Verification items for the finished model (mm, model axes). Face numbers are marked on the shaded views. A direction names the side the tool comes from. Round coordinates to 2 decimals unless told otherwise and drop trailing zeros. Order: outer loops, then holes, each group sorted by start corner. A loop starts at its lowest first (then second) coordinate and runs counter-clockwise, first axis right, second up. Notation, with made-up numbers: M 81.25,61.25 L 91.25,61.25 A27 cw 91.25,92.25 Z; hole C -22.75,-25 d10. An arc over 180 degrees is marked long. Use CSV: the item, a comma, the result in double quotes. Start each with the question number.
Q1. Set-up check for the marked faces 5, 6 and 7: record each of +Z, -Z, +X, -X, +Y, -Y from which the full face is reachable in a straight line by a thin tool's end or side.
Q2. Sectioned sample at B-B (x = 41). Enter the section's corners in (y, z), and give its area (3 significant figures).
Q3. Sectioned sample at C-C (z = 6). Enter the section's corners in (x, y) (3 decimals), and give its area (3 significant figures).
Q4. Mould release check, pull along X, two halves, no side actions. Record for the marked faces 1, 2, 3 and 4: +X half, -X half, draft (parallel to the pull), parting line (faces both ways), or undercut.
Q5. Sectioned sample at D-D (y = 43). Enter the section's corners in (x, z).
Q6. Sectioned sample at A-A (y = 17). Enter the section's corners in (x, z) (3 decimals).
Q7. Scan lines: line 1 (Z direction, x = -88, y = 8.5); line 2 (Z direction, x = -26.5, y = 17); line 3 (X direction, y = -8.5, z = 23). Record each from-to range of solid material in increasing order.
Q8. Gauge pin test, flat ends, axial feed: pin 1 Ø12 at (x, z) = (-36, 21.5) entering from +Y; pin 2 Ø0.6 at (x, z) = (98, 33) entering from +Y; pin 3 Ø1.5 at (x, z) = (60.5, 18.5) entering from +Y. Record the tip position at first contact, or that the pin passes through.
```python
from build123d import *

# Parameters (mm, degrees)
SKETCH2_W                = 198
SKETCH2_H                = 78
BOSS_EXTRUDE1_DEPTH      = 50
BOSS_EXTRUDE1_DEPTH_BACK = 15
SHELL1_T                 = -2
BOSS_EXTRUDE2_REACH      = 198
SKETCH3_W                = 2.5
SKETCH3_H                = 2
CUT_EXTRUDE1_REACH       = 4
CROQUIS1_W               = 35.265
CROQUIS1_H               = 26
SALIENTE_EXTRUIR1_DEPTH  = 38.9
CORTAR_EXTRUIR1_DEPTH    = 2
CORTAR_EXTRUIR2_DEPTH    = 30
CROQUIS5_W               = 26
CROQUIS5_H               = 15
CORTAR_EXTRUIR3_DEPTH    = 35.265
CROQUIS6_W               = 12
CROQUIS6_H               = 3
SALIENTE_EXTRUIR2_DEPTH  = 3
CROQUIS7_W               = 26
CROQUIS7_H               = 15
CORTAR_EXTRUIR4_DEPTH    = 35.265


with BuildPart() as part:
    # Sketch2 → Boss-Extrude1 (new body, two sides)
    with BuildSketch(Plane(origin=(0, 0, 0), x_dir=(1, 0, 0), z_dir=(0, 1, 0))) as boss_extrude1_sk:
        Rectangle(SKETCH2_W, SKETCH2_H)
    extrude(amount=BOSS_EXTRUDE1_DEPTH)
    extrude(boss_extrude1_sk.sketch, amount=-BOSS_EXTRUDE1_DEPTH_BACK)

    # Shell1
    shell1_openings = [part.faces().sort_by_distance(p)[0] for p in [
        (0, 50, 0),
    ]]
    offset(amount=SHELL1_T, openings=shell1_openings, kind=Kind.INTERSECTION)

    # Sketch3 → Boss-Extrude2 (add, up to next)
    with BuildSketch(Plane(origin=(-97, 0, 0), x_dir=(0, 0, -1), z_dir=(1, 0, 0)), mode=Mode.PRIVATE) as boss_extrude2_sk1:
        with Locations((-35.75, 49)):
            Rectangle(SKETCH3_W, SKETCH3_H)
    boss_extrude2_tool1 = extrude(boss_extrude2_sk1.sketch, amount=BOSS_EXTRUDE2_REACH, mode=Mode.PRIVATE) - part.part
    add(boss_extrude2_tool1.solids().sort_by_distance((-97, 49, 35.75))[0])
    # Sketch3 → Boss-Extrude2 (add, up to next)
    with BuildSketch(Plane(origin=(-97, 0, 0), x_dir=(0, 0, -1), z_dir=(1, 0, 0)), mode=Mode.PRIVATE) as boss_extrude2_sk2:
        with Locations((35.75, 49)):
            Rectangle(SKETCH3_W, SKETCH3_H)
    boss_extrude2_tool2 = extrude(boss_extrude2_sk2.sketch, amount=BOSS_EXTRUDE2_REACH, mode=Mode.PRIVATE) - part.part
    add(boss_extrude2_tool2.solids().sort_by_distance((-97, 49, -35.75))[0])

    # Sketch4 → Cut-Extrude1 (cut, up to next)
    with BuildSketch(Plane.ZY.offset(-97), mode=Mode.PRIVATE) as cut_extrude1_sk1:
        Polygon((-37, 48), (-37, 45), (-31.5, 45), (-31.5, 50), (-34.5, 50), (-34.5, 48), align=None)
    cut_extrude1_tool1 = extrude(cut_extrude1_sk1.sketch, amount=-CUT_EXTRUDE1_REACH, mode=Mode.PRIVATE) & part.part
    add(cut_extrude1_tool1.solids().sort_by_distance((97, 47.166667, -33.916667))[0], mode=Mode.SUBTRACT)
    # Sketch4 → Cut-Extrude1 (cut, up to next)
    with BuildSketch(Plane.ZY.offset(-97), mode=Mode.PRIVATE) as cut_extrude1_sk2:
        Polygon((34.5, 48), (37, 48), (37, 45), (31.5, 45), (31.5, 50), (34.5, 50), align=None)
    cut_extrude1_tool2 = extrude(cut_extrude1_sk2.sketch, amount=-CUT_EXTRUDE1_REACH, mode=Mode.PRIVATE) & part.part
    add(cut_extrude1_tool2.solids().sort_by_distance((97, 47.166667, 33.916667))[0], mode=Mode.SUBTRACT)

    # Croquis1 → Saliente-Extruir1 (add)
    with BuildSketch(Plane(origin=(0, -13, 0), x_dir=(1, 0, 0), z_dir=(0, 1, 0))):
        with Locations((79.3675, -16.5)):
            Rectangle(CROQUIS1_W, CROQUIS1_H)
    saliente_extruir1 = extrude(amount=SALIENTE_EXTRUIR1_DEPTH)

    # Simetría1: Saliente-Extruir1 across plane
    add(saliente_extruir1.mirror(Plane(origin=(0, 0, 0), x_dir=(0, 0, 1), z_dir=(1, 0, 0))))

    # Croquis2 → Cortar-Extruir1 (cut)
    with BuildSketch(Plane(origin=(0, 25.9, 0), x_dir=(1, 0, 0), z_dir=(0, 1, 0))):
        with BuildLine():
            Line((82.41, -12.375), (82.41, -20.625))
            ThreePointArc((82.41, -20.625), (79.235, -23.8), (76.06, -20.625))
            Line((76.06, -20.625), (76.06, -12.375))
            ThreePointArc((76.06, -12.375), (79.235, -9.2), (82.41, -12.375))
        make_face()
    cortar_extruir1 = extrude(amount=-CORTAR_EXTRUIR1_DEPTH, mode=Mode.SUBTRACT)

    # Simetría2: Cortar-Extruir1 across plane
    add(cortar_extruir1.mirror(Plane(origin=(0, 0, 0), x_dir=(0, 0, 1), z_dir=(1, 0, 0))), mode=Mode.SUBTRACT)

    # Croquis3 → Cortar-Extruir2 (cut)
    with BuildSketch(Plane(origin=(0, 23.9, 0), x_dir=(1, 0, 0), z_dir=(0, 1, 0))):
        with BuildLine():
            Line((80.835, -13.2), (80.835, -19.8))
            ThreePointArc((80.835, -19.8), (79.235, -21.4), (77.635, -19.8))
            Line((77.635, -19.8), (77.635, -13.2))
            ThreePointArc((77.635, -13.2), (79.235, -11.6), (80.835, -13.2))
        make_face()
    cortar_extruir2 = extrude(amount=-CORTAR_EXTRUIR2_DEPTH, mode=Mode.SUBTRACT)

    # Simetría3: Cortar-Extruir2 across plane
    add(cortar_extruir2.mirror(Plane(origin=(0, 0, 0), x_dir=(0, 0, 1), z_dir=(1, 0, 0))), mode=Mode.SUBTRACT)

    # Croquis5 → Cortar-Extruir3 (cut)
    with BuildSketch(Plane.ZY.offset(-61.735)):
        with Locations((16.5, -5.5)):
            Rectangle(CROQUIS5_W, CROQUIS5_H)
    extrude(amount=-CORTAR_EXTRUIR3_DEPTH, mode=Mode.SUBTRACT)

    # Croquis6 → Saliente-Extruir2 (add)
    with BuildSketch(Plane.ZY.offset(-61.735)):
        with Locations((16.5, 3.5)):
            Rectangle(CROQUIS6_W, CROQUIS6_H)
    saliente_extruir2 = extrude(amount=SALIENTE_EXTRUIR2_DEPTH)

    # Croquis7 → Cortar-Extruir4 (cut)
    with BuildSketch(Plane(origin=(-61.735, 0, 0), x_dir=(0, 0, -1), z_dir=(1, 0, 0))):
        with Locations((-16.5, -5.5)):
            Rectangle(CROQUIS7_W, CROQUIS7_H)
    extrude(amount=-CORTAR_EXTRUIR4_DEPTH, mode=Mode.SUBTRACT)

    # Simetría7: Saliente-Extruir2 across plane
    add(saliente_extruir2.mirror(Plane(origin=(0, 0, 0), x_dir=(0, 0, 1), z_dir=(1, 0, 0))))


solid = part.part
```
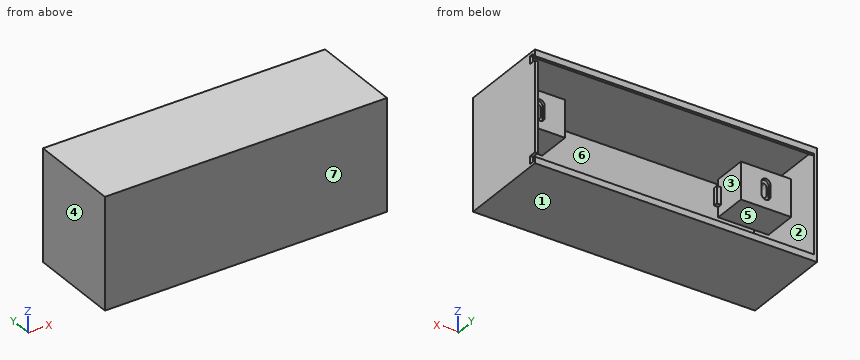
Verdict:
1,face 5,"+Y"
1,face 6,"none"
1,face 7,"+Z, -Z, +X, -X, -Y"
2,outline,"M -15,-39 L 50,-39 L 50,-34.5 L 48,-34.5 L 48,-37 L -13,-37 L -13,37 L 48,37 L 48,34.5 L 50,34.5 L 50,39 L -15,39 Z"
2,area,"418 mm²"
3,outline,"M -99,-15 L 99,-15 L 99,50 L 97,50 L 97,25.9 L 61.735,25.9 L 61.735,2 L 97,2 L 97,-13 L -97,-13 L -97,2 L -61.735,2 L -61.735,25.9 L -97,25.9 L -97,50 L -99,50 Z"
3,area,"2,330 mm²"
4,face 1,"draft"
4,face 2,"undercut"
4,face 3,"undercut"
4,face 4,"-X half"
5,outline,"M -99,-39 L 99,-39 L 99,39 L -99,39 Z; hole M -97,-37 L 97,-37 L 97,37 L -97,37 Z"
6,outline,"M -99,-39 L 99,-39 L 99,39 L -99,39 Z; hole M -97,-37 L 97,-37 L 97,3.5 L 61.735,3.5 L 61.735,29.5 L 97,29.5 L 97,37 L -97,37 L -97,29.5 L -61.735,29.5 L -61.735,3.5 L -97,3.5 Z; hole M -80.835,13.2 A1.6 ccw -77.635,13.2 L -77.635,19.8 A1.6 ccw -80.835,19.8 Z; hole M 77.635,13.2 A1.6 ccw 80.835,13.2 L 80.835,19.8 A1.6 ccw 77.635,19.8 Z"
7,line 1,"z = -39 to -37, 3.5 to 29.5, 37 to 39"
7,line 2,"z = -39 to -37, 37 to 39"
7,line 3,"x = -99 to -97, 97 to 99"
8,pin 1,"stops at y = -13"
8,pin 2,"stops at y = 45"
8,pin 3,"stops at y = 5"
